Read the model definition and answer for the solid it produces. Units are mm, in the model's axes. A direction names the side the tool comes from. Give positions to 0.01 mm unless a question says otherwise; leave off trailing zeros. Order: outer loops, then holes, each group sorted by start corner. A loop starts at its lowest first (then second) coordinate and runs counter-clockwise, first axis right, second up. Notation, with made-up numbers: (-29.5, 28) - (-20.5, 28) arc R10 ccw to (-20.5, 43) - close; hole circle Ø5 at (-30.5, 44.5). An arc over 180 degrees is marked (long way). Return JSON: item names as keys, results as strings.
```python
from build123d import *

# Parameters (mm, degrees)
F0_W      = 2
F0_H      = 10
F0_H_2    = 15
F1_DEPTH  = 15
F2_W      = 15
F2_H      = 15
F3_DEPTH  = 65
F5_DEPTH  = 25
F6_DEPTH  = 5
F7_R      = 2.875
F8_DEPTH  = 5
F9_DEPTH  = 25
F10_W     = 10
F10_H     = 3.7
F10_W_2   = 7.5
F11_DEPTH = 25
F12_W     = 30.5
F12_H     = 15
F13_DEPTH = 2
F14_R     = 1.75


with BuildPart() as f1:
    # F0 (on Top) → F1 (new body)
    with BuildSketch(Plane.XY):
        with Locations((-25.5, -71.0108693689)):
            Rectangle(F0_W, F0_H)
        Polygon((31, 3.9891306311), (-30, 3.9891306311), (-30, -91.0108693689), (-26.5, -91.0108693689), (-26.5, -76.0108693689), (-26.5, -66.0108693689), (-26.5, 0.4891306311), (27.5, 0.4891306311), (27.5, -11.0108693689), (21.5, -11.0108693689), (21.5, -15.0108693689), (31, -15.0108693689), align=None)
        with Locations((-25.5, -83.5108693689)):
            Rectangle(F0_W, F0_H_2)
    extrude(amount=F1_DEPTH)

    # F2 (on face) → F3 (join)
    with BuildSketch(Plane(origin=(-30, 0, 0), x_dir=(0, -1, 0), z_dir=(-1, 0, 0))):
        with Locations((83.5108693689, 7.5)):
            Rectangle(F2_W, F2_H)
    extrude(amount=F3_DEPTH)

    # F4 (on face) → F5 (cut)
    with BuildSketch(Plane.XY.offset(15)):
        with BuildLine():
            ThreePointArc((-95, -83.5108693689), (-92.8033008589, -78.20756851), (-87.5, -76.0108693689))
            Line((-87.5, -76.0108693689), (-95, -76.0108693689))
            Line((-95, -76.0108693689), (-95, -83.5108693689))
        make_face()
        with BuildLine():
            Line((-95, -91.0108693689), (-87.5, -91.0108693689))
            ThreePointArc((-87.5, -91.0108693689), (-92.8033008589, -88.8141702278), (-95, -83.5108693689))
            Line((-95, -83.5108693689), (-95, -91.0108693689))
        make_face()
    extrude(amount=-F5_DEPTH, mode=Mode.SUBTRACT)

    # F4 (on face) → F6 (join)
    with BuildSketch(Plane.XY.offset(15)):
        with BuildLine():
            ThreePointArc((-80, -83.5108693689), (-82.1966991411, -78.20756851), (-87.5, -76.0108693689))
            ThreePointArc((-87.5, -76.0108693689), (-92.8033008589, -78.20756851), (-95, -83.5108693689))
            ThreePointArc((-95, -83.5108693689), (-92.8033008589, -88.8141702278), (-87.5, -91.0108693689))
            ThreePointArc((-87.5, -91.0108693689), (-82.1966991411, -88.8141702278), (-80, -83.5108693689))
        make_face()
        with BuildLine():
            ThreePointArc((-84.625, -83.5108693689), (-87.5, -86.3858693689), (-90.375, -83.5108693689))
            ThreePointArc((-90.375, -83.5108693689), (-87.5, -80.6358693689), (-84.625, -83.5108693689))
        make_face(mode=Mode.SUBTRACT)
    extrude(amount=F6_DEPTH)

    # F7 (on face) → F8 (cut)
    with BuildSketch(Plane.XY.offset(20)):
        Polygon((-85, -79.18074235), (-90, -79.18074235), (-92.5, -83.5108693689), (-90, -87.8409963878), (-85, -87.8409963878), (-82.5, -83.5108693689), align=None)
        with Locations((-87.5, -83.5108693689)):
            Circle(F7_R, mode=Mode.SUBTRACT)
    extrude(amount=-F8_DEPTH, mode=Mode.SUBTRACT)

    # F4 (on face) → F9 (cut)
    with BuildSketch(Plane.XY.offset(15)):
        with BuildLine():
            ThreePointArc((-84.625, -83.5108693689), (-87.5, -80.6358693689), (-90.375, -83.5108693689))
            ThreePointArc((-90.375, -83.5108693689), (-87.5, -86.3858693689), (-84.625, -83.5108693689))
        make_face()
    extrude(amount=-F9_DEPTH, mode=Mode.SUBTRACT)

    # F10 (on face) → F11 (cut)
    with BuildSketch(Plane.XZ.offset(91.0108693689)):
        with Locations((-75, 10.75)):
            Rectangle(F10_W, F10_H)
        with Locations((-91.25, 10.75)):
            Rectangle(F10_W_2, F10_H)
        with Locations((-83.75, 10.75)):
            Rectangle(F10_W_2, F10_H)
        with Locations((-83.75, 4.25)):
            Rectangle(F10_W_2, F10_H)
        with Locations((-91.25, 4.25)):
            Rectangle(F10_W_2, F10_H)
        with Locations((-75, 4.25)):
            Rectangle(F10_W, F10_H)
    extrude(amount=-F11_DEPTH, mode=Mode.SUBTRACT)

    # F12 (on face) → F13 (join)
    with BuildSketch(Plane.YZ.offset(-26.5)):
        with Locations((-50.7608693689, 7.5)):
            Rectangle(F12_W, F12_H)
    extrude(amount=F13_DEPTH)

    # F14
    f14_edges = [f1.edges().sort_by_distance(p)[0] for p in [
        (-30, -76.010869, 7.5),
        (-30, 3.989131, 7.5),
        (31, 3.989131, 7.5),
        (31, -15.010869, 7.5),
        (21.5, -15.010869, 7.5),
        (-24.5, -91.010869, 7.5),
    ]]
    fillet(f14_edges, radius=F14_R)


solid = f1.part
```
Q1. Given pin 1 (4.5 mm diameter, centred on x = -87.5, y = -83.51, fed in from -Z); pin 2 (8 mm diameter, centred on x = -61.5, z = 9.5, fed in from +Y); pin 3 (1.5 mm diameter, centred on y = -33, z = 7, fed in from -X); pin 4 (1.9 mm diameter, centred on y = -84.5, z = 5, fed in from -X), each flat-ended and moving along its own axis, determine where each tip first touches the part or whether it passes through.
Values:
{"pin 1": "passes through", "pin 2": "stops at y = -76.01", "pin 3": "stops at x = -30", "pin 4": "stops at x = -70"}
Q2. Determine the mould class of faces 4 (the flat face through (-83.77, -85.71, 17.54)), 5 (the flat face through (-28, -58, 0)), 6 (the flat face through (-70, -84, 4)) for opening direction Z: released by +Z, released by -Z, zero draft, split by the parting line, or undercut.
Values:
{"face 4": "zero draft", "face 5": "released by -Z", "face 6": "undercut"}
Q3. A cutting plane is placed at D-D (z = 17). Write down the section's boundary in (x, y).
Values:
{"outline": "circle Ø15 at (-87.5, -83.51); hole (-92.5, -83.51) - (-90, -87.84) - (-85, -87.84) - (-82.5, -83.51) - (-85, -79.18) - (-90, -79.18) - close"}
Q4. A cutting plane is placed at C-C (y = -50.5). Write down the section's boundary in (x, z).
Values:
{"outline": "(-30, 0) - (-24.5, 0) - (-24.5, 15) - (-30, 15) - close"}
Q5. For faces 1 (the flat face through (-30, -35, 7)), 2 (the flat face through (-83, -84, 2.4)), 3 (the flat face through (25, -11.011, 7)), determine the directions among +Z, -Z, +X, -X, +Y, -Y from which every point of the face is accessible in a straight line to the end or side of a thin tool.
Values:
{"face 1": "+Z, -Z, -X, +Y", "face 2": "-X, +Y, -Y", "face 3": "+Z, -Z"}
Q6. A cutting plane is placed at A-A (x = -72.5). Write down the section's boundary in (y, z).
Values:
{"outline": "(-91.01, 0) - (-76.01, 0) - (-76.01, 2.4) - (-91.01, 2.4) - close; (-91.01, 6.1) - (-76.01, 6.1) - (-76.01, 8.9) - (-91.01, 8.9) - close; (-91.01, 12.6) - (-76.01, 12.6) - (-76.01, 15) - (-91.01, 15) - close"}
Q7. A cutting plane is placed at B-B (z = 7.5). Write down the section's boundary in (x, y) (3 decimals), and give its area (3 significant figures).
Values:
{"outline": "(-87.5, -91.011) - (-26.25, -91.011) arc R1.75 ccw to (-24.5, -89.261) - (-24.5, -35.511) - (-26.5, -35.511) - (-26.5, 0.489) - (27.5, 0.489) - (27.5, -11.011) - (21.5, -11.011) - (21.5, -13.261) arc R1.75 ccw to (23.25, -15.011) - (29.25, -15.011) arc R1.75 ccw to (31, -13.261) - (31, 2.239) arc R1.75 ccw to (29.25, 3.989) - (-28.25, 3.989) arc R1.75 ccw to (-30, 2.239) - (-30, -74.261) arc R1.75 cw to (-31.75, -76.011) - (-87.5, -76.011) arc R7.5 ccw to start; hole circle Ø5.75 at (-87.5, -83.511)", "area": "1,650 mm²"}
Q8. Consider L1, parallel to Z at x = -85.5, y = -81; L2, parallel to Y at x = -87.5, z = 14.5; L3, parallel to X at y = -0.5, z = 8.5. Determine where each line is inside the solid, lowest interval first.
Values:
{"L1": "z = 0 to 2.4, 6.1 to 8.9, 12.6 to 15", "L2": "y = -91.01 to -86.39, -80.64 to -76.01", "L3": "x = -30 to -26.5, 27.5 to 31"}
